Verification items for the finished model (mm, model axes). Round coordinates to 2 decimals unless told otherwise and drop trailing zeros. Order: outer loops, then holes, each group sorted by start corner. A loop starts at its lowest first (then second) coordinate and runs counter-clockwise, first axis right, second up.
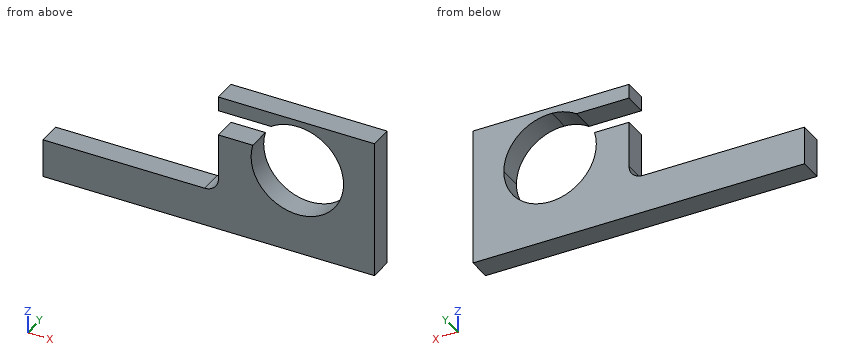
```python
from build123d import *

# Parameters (mm, degrees)
F0_W     = 273.05
F0_H     = 114.3
F1_DEPTH = 19.05
F3_DEPTH = 25.4
F5_DEPTH = 25.4


with BuildPart() as f1:
    # F0 (on Front) → F1 (new body)
    with BuildSketch(Plane.XZ):
        with Locations((136.525, 57.15)):
            Rectangle(F0_W, F0_H)
    extrude(amount=F1_DEPTH)

    # F2 (on Front) → F3 (cut)
    with BuildSketch(Plane.XZ):
        with BuildLine():
            Line((144.5167429344, 115.0370560134), (0, 114.3))
            Line((0, 114.3), (0, 31.75))
            Line((0, 31.75), (133.0867429344, 31.75))
            ThreePointArc((133.0867429344, 31.75), (141.1689734434, 35.097769491), (144.5167429344, 43.18))
            Line((144.5167429344, 43.18), (144.5167429344, 82.55))
            Line((144.5167429344, 82.55), (157.2167429344, 82.55))
            Line((157.2167429344, 82.55), (157.2167429344, 102.3370560134))
            Line((157.2167429344, 102.3370560134), (144.5167429344, 102.3370560134))
            Line((144.5167429344, 102.3370560134), (144.5167429344, 115.0370560134))
        make_face()
    extrude(amount=F3_DEPTH, mode=Mode.SUBTRACT)

    # F4 (on Front) → F5 (cut)
    with BuildSketch(Plane.XZ):
        with BuildLine():
            ThreePointArc((172.8805950089, 81.4623758197), (204.3295752166, 33.3793433406), (247.65, 71.12))
            ThreePointArc((247.65, 71.12), (235.9531055724, 98.5879088416), (208.0444348487, 109.1902413123))
            ThreePointArc((208.0444348487, 109.1902413123), (197.4832243591, 107.2586624771), (187.8802183492, 102.4573668838))
            Line((187.8802183492, 102.4573668838), (192.520737648, 102.4573668838))
            Line((192.520737648, 102.4573668838), (192.520737648, 81.4623758197))
            Line((192.520737648, 81.4623758197), (172.8805950089, 81.4623758197))
        make_face()
        with BuildLine():
            Line((144.0413892269, 81.4623758197), (172.8805950089, 81.4623758197))
            ThreePointArc((172.8805950089, 81.4623758197), (178.5489905494, 93.26830497), (187.8802183492, 102.4573668838))
            Line((187.8802183492, 102.4573668838), (156.6383838654, 102.4573668838))
            Line((156.6383838654, 102.4573668838), (144.0413892269, 102.4573668838))
            Line((144.0413892269, 102.4573668838), (144.0413892269, 81.4623758197))
        make_face()
        with BuildLine():
            ThreePointArc((187.8802183492, 102.4573668838), (178.5489905494, 93.26830497), (172.8805950089, 81.4623758197))
            Line((172.8805950089, 81.4623758197), (192.520737648, 81.4623758197))
            Line((192.520737648, 81.4623758197), (192.520737648, 102.4573668838))
            Line((192.520737648, 102.4573668838), (187.8802183492, 102.4573668838))
        make_face()
    extrude(amount=F5_DEPTH, mode=Mode.SUBTRACT)


solid = f1.part
```
1) Sectioned sample at C-C on x = 47. Record the cut outline in (y, z).
2) Scan lines: probe 1 along Z at (x, y) = (209.55, -8.75); probe 2 along Z at (x, y) = (151, -11); probe 3 along X at (y, z) = (-13, 71.12). Record each from-to range of solid material in increasing order.
3) Sectioned sample at B-B on z = 46.5. Record the cut outline in (x, y), then the cut area to 3 significant figures.
4) Sectioned sample at A-A on y = -8.25. Record the cut outline in (x, z).
5) Go/stop test with a flat-tipped pin: pin 1 Ø9.5 at (y, z) = (-6.5, 108) entering from -X. Record where the tip stops, or that it passes through.
Returned:
1. outline: (-19.05, 0) - (0, 0) - (0, 31.75) - (-19.05, 31.75) - close
2. probe 1: z = 0 to 33.02, 109.22 to 114.3
2. probe 2: z = 0 to 81.46, 102.46 to 114.3
2. probe 3: x = 144.52 to 171.45, 247.65 to 273.05
3. outline: (144.52, -19.05) - (180.47, -19.05) - (180.47, 0) - (144.52, 0) - close; (238.63, -19.05) - (273.05, -19.05) - (273.05, 0) - (238.63, 0) - close
3. area: 1,340 mm2
4. outline: (0, 0) - (273.05, 0) - (273.05, 114.3) - (144.52, 114.3) - (144.52, 102.46) - (187.88, 102.46) arc R38.1 cw (long way) to (172.88, 81.46) - (144.52, 81.46) - (144.52, 43.18) arc R11.43 cw to (133.09, 31.75) - (0, 31.75) - close
5. pin 1: stops at x = 144.52
